Check sheet for the modelled part. Datum: model origin and axes. Units: mm. A direction names the side the tool comes from. Coordinates: 2 decimals unless noted, no trailing zeros. Loops run counter-clockwise (first coordinate to the right, second up) from the corner with the lowest first, then second, coordinate; pieces in that order, holes last. Notation, with made-up numbers: M -22,38.25 L 20,38.25 A31 cw 20,76.25 Z; hole C 15.5,-36 d10. An arc over 180 degrees is marked long. Answer in a Markdown table with one row per item. Add a question column.
```python
from build123d import *

# Parameters (mm, degrees)
SKETCH3_W            = 55.1053
SKETCH3_H            = 45.5803
BOSS_EXTRUDE2_DEPTH  = 44.45
SKETCH11_W           = 51.1175
SKETCH11_H           = 41.5925
SKETCH11_W_2         = 47.9425
SKETCH11_H_2         = 38.4175
BOSS_EXTRUDE3_DEPTH  = 3.175
SKETCH13_W           = 44.7675
SKETCH13_H           = 35.2425
CUT_EXTRUDE3_DEPTH   = 73.294764944
CUT_EXTRUDE4_DEPTH   = 5.1689
SKETCH19_W           = 1.5875
SKETCH19_H           = 45.5803
BOSS_EXTRUDE4_DEPTH  = 44.45
SKETCH21_W           = 1.905
SKETCH21_H           = 35.2425
CUT_EXTRUDE5_DEPTH   = 39.37
FILLET1_R            = 406.4
FILLET2_R            = 406.4
SKETCH22_R           = 1.524
CUT_EXTRUDE7_DEPTH   = 3.175
BOSS_EXTRUDE5_DEPTH  = 38.1
SKETCH39_R           = 1.296908885
SKETCH39_R_2         = 1.27
CUT_EXTRUDE14_DEPTH  = 25.4
BOSS_EXTRUDE22_DEPTH = 8.89
CUT_EXTRUDE15_DEPTH  = 88.778493945
SKETCH48_W           = 18.8595
SKETCH48_H           = 29.21
BOSS_EXTRUDE23_DEPTH = 1.5875
SKETCH52_R           = 1.27
CUT_EXTRUDE16_DEPTH  = 25.4


with BuildPart() as part:
    # Sketch3 → Boss-Extrude2 (new body)
    with BuildSketch(Plane(origin=(0, 0, 0), x_dir=(1, 0, 0), z_dir=(0, 1, 0))):
        with Locations((6.69887245, -22.79015)):
            Rectangle(SKETCH3_W, SKETCH3_H)
    extrude(amount=BOSS_EXTRUDE2_DEPTH)

    # Sketch11 → Boss-Extrude3 (add)
    with BuildSketch(Plane(origin=(0, 44.45, 0), x_dir=(1, 0, 0), z_dir=(0, 1, 0))):
        with Locations((6.69887245, -22.79015)):
            Rectangle(SKETCH11_W, SKETCH11_H)
        with Locations((6.69887245, -22.79015)):
            Rectangle(SKETCH11_W_2, SKETCH11_H_2, mode=Mode.SUBTRACT)
    extrude(amount=BOSS_EXTRUDE3_DEPTH)

    # Sketch13 → Cut-Extrude3 (cut, through all)
    with BuildSketch(Plane(origin=(0, 44.45, 0), x_dir=(1, 0, 0), z_dir=(0, 1, 0))):
        with Locations((6.69887245, -22.79015)):
            Rectangle(SKETCH13_W, SKETCH13_H)
    extrude(amount=-CUT_EXTRUDE3_DEPTH, mode=Mode.SUBTRACT)

    # Sketch14 → Cut-Extrude4 (cut)
    with BuildSketch(Plane.XY.offset(45.5803)):
        with BuildLine():
            Line((-2.82612755, 6.35), (-2.82612755, 0))
            Line((-2.82612755, 0), (3.52387245, 0))
            Line((3.52387245, 0), (3.52387245, 6.35))
            ThreePointArc((3.52387245, 6.35), (0.34887245, 9.525), (-2.82612755, 6.35))
        make_face()
        with BuildLine():
            Line((9.87387245, 6.35), (9.87387245, 0))
            Line((9.87387245, 0), (16.22387245, 0))
            Line((16.22387245, 0), (16.22387245, 6.35))
            ThreePointArc((16.22387245, 6.35), (13.04887245, 9.525), (9.87387245, 6.35))
        make_face()
        with BuildLine():
            Line((26.465313364, 0), (30.581222486, 0))
            Line((30.581222486, 0), (30.581222486, 6.35))
            ThreePointArc((30.581222486, 6.35), (28.523267925, 8.407954561), (26.465313364, 6.35))
            Line((26.465313364, 6.35), (26.465313364, 0))
        make_face()
    extrude(amount=-CUT_EXTRUDE4_DEPTH, mode=Mode.SUBTRACT)

    # Sketch19 → Boss-Extrude4 (add)
    with BuildSketch(Plane.XZ):
        with Locations((-21.64752755, 22.79015)):
            Rectangle(SKETCH19_W, SKETCH19_H)
        with Locations((35.04527245, 22.79015)):
            Rectangle(SKETCH19_W, SKETCH19_H)
    extrude(amount=-BOSS_EXTRUDE4_DEPTH)

    # Sketch21 → Cut-Extrude5 (cut)
    with BuildSketch(Plane(origin=(0, 0, 0), x_dir=(-1, 0, 0), z_dir=(0, -1, 0))):
        with Locations((16.63737755, -22.79015)):
            Rectangle(SKETCH21_W, SKETCH21_H)
        with Locations((-30.03512245, -22.79015)):
            Rectangle(SKETCH21_W, SKETCH21_H)
    extrude(amount=-CUT_EXTRUDE5_DEPTH, mode=Mode.SUBTRACT)

    # Fillet1
    # the kernel refuses this fillet: 406.4 mm, written as the material it adds along each edge
    with BuildSketch(Plane(origin=(-17.58987755, 39.37, 40.4114), x_dir=(0, -1, 0), z_dir=(0, 0, -1))) as fillet1_piece_1:
        with BuildLine():
            CenterArc((39.303371039, -406.4), FILLET1_R, 90, 5.549809332)
            Line((0, -1.905), (0, 0))
            Line((0, 0), (39.303371039, 0))
        make_face()
    extrude(amount=35.2425)

    # Fillet2
    # the kernel refuses this fillet: 406.4 mm, written as the material it adds along each edge
    with BuildSketch(Plane(origin=(30.98762245, 39.37, -93.089527597), x_dir=(-1, 0, 0), z_dir=(0, 0, 1))) as fillet2_piece_1_section:
        with BuildLine():
            CenterArc((406.4, 39.303371039), FILLET2_R, 180, 5.549809332)
            Line((0, 39.303371039), (0, 0))
            Line((0, 0), (1.905, 0))
        make_face()
    fillet2_piece_1 = extrude(amount=231.759355193, mode=Mode.PRIVATE)
    fillet2_piece_1 = split(fillet2_piece_1, bisect_by=Plane(origin=(30.98762245, 39.37, 45.5803), z_dir=(0, 0, -1)), keep=Keep.TOP, mode=Mode.PRIVATE)
    fillet2_piece_1 = split(fillet2_piece_1, bisect_by=Plane(origin=(30.98762245, 39.37, 0), z_dir=(0, 0, 1)), keep=Keep.TOP, mode=Mode.PRIVATE)
    add(fillet2_piece_1)

    # Sketch22 → Cut-Extrude7 (cut)
    with BuildSketch(Plane.XZ):
        with Locations(Location((-19.64727755, 42.7863, 0), (0, 0, 270))):
            Circle(SKETCH22_R)
        with Locations(Location((33.04502245, 42.7863, 0), (0, 0, 270))):
            Circle(SKETCH22_R)
        with Locations(Location((-19.64727755, 2.794, 0), (0, 0, 270))):
            Circle(SKETCH22_R)
        with Locations(Location((33.04502245, 2.794, 0), (0, 0, 270))):
            Circle(SKETCH22_R)
    extrude(amount=-CUT_EXTRUDE7_DEPTH, mode=Mode.SUBTRACT)

    # Sketch23 → Boss-Extrude5 (add)
    with BuildSketch(Plane.XZ):
        with BuildLine():
            Line((22.13572245, 62.8523), (22.13572245, 64.4398))
            Line((22.13572245, 64.4398), (21.379894456, 64.4398))
            Line((21.379894456, 64.4398), (-12.40827755, 64.4398))
            add(Edge.make_bspline(
                [(-12.40827755, 64.4398), (-22.44127755, 64.4398), (-22.44127755, 45.5803)],
                knots=[0, 0, 0, 1.570796327, 1.570796327, 1.570796327], degree=2, weights=[1, 0.707106781, 1]))
            Line((-22.44127755, 45.5803), (-11.13827755, 45.5803))
            Line((-11.13827755, 45.5803), (-11.13827755, 58.170091836))
            Line((-11.13827755, 58.170091836), (-11.13827755, 62.8523))
            Line((-11.13827755, 62.8523), (22.13572245, 62.8523))
        make_face()
    extrude(amount=-BOSS_EXTRUDE5_DEPTH)

    # Sketch39 → Cut-Extrude14 (cut)
    with BuildSketch(Plane.XY.offset(64.4398)):
        with Locations((5.46697245, 34.925)):
            Circle(SKETCH39_R)
        with Locations((-10.02702755, 34.925)):
            Circle(SKETCH39_R_2)
        with Locations((20.96097245, 34.925)):
            Circle(SKETCH39_R_2)
    extrude(amount=-CUT_EXTRUDE14_DEPTH, mode=Mode.SUBTRACT)

    # Sketch43 → Boss-Extrude22 (add)
    with BuildSketch(Plane.XZ):
        with BuildLine():
            Line((30.58122245, 45.5803), (35.83902245, 45.5803))
            add(Edge.make_bspline(
                [(35.83902245, 45.5803), (35.83902245, 63.254133988), (24.53602245, 64.4398)],
                knots=[4.71238898, 4.71238898, 4.71238898, 6.216048931, 6.216048931, 6.216048931], degree=2, weights=[1, 0.730440262, 1]))
            Line((24.53602245, 64.4398), (22.13572245, 64.4398))
            Line((22.13572245, 64.4398), (22.13572245, 45.5803))
            Line((22.13572245, 45.5803), (23.72322245, 45.5803))
            Line((23.72322245, 45.5803), (23.72322245, 58.7883))
            Line((23.72322245, 58.7883), (30.58122245, 58.7883))
            Line((30.58122245, 58.7883), (30.58122245, 45.5803))
        make_face()
    extrude(amount=-BOSS_EXTRUDE22_DEPTH)

    # Sketch51 → Cut-Extrude15 (cut, through all)
    with BuildSketch(Plane.XY.offset(64.4398)):
        with BuildLine():
            add(Edge.make_bspline(
                [(-20.85377755, 44.45), (-22.44127755, 44.45), (-22.44127755, 8.89)],
                knots=[3.141592654, 3.141592654, 3.141592654, 4.71238898, 4.71238898, 4.71238898], degree=2, weights=[1, 0.707106781, 1]))
            Line((-22.44127755, 8.89), (-23.728758276, 8.89))
            Line((-23.728758276, 8.89), (-23.728758276, 45.620970636))
            Line((-23.728758276, 45.620970636), (-20.85377755, 45.620970636))
            Line((-20.85377755, 45.620970636), (-20.85377755, 44.45))
        make_face()
        with BuildLine():
            add(Edge.make_bspline(
                [(35.83902245, 8.89), (35.83902245, 34.352534387), (34.251533964, 44.439253731)],
                knots=[4.71238898, 4.71238898, 4.71238898, 5.875876601, 5.875876601, 5.875876601], degree=2, weights=[1, 0.835505729, 1]))
            Line((34.251533964, 44.439253731), (34.25152245, 44.45))
            Line((34.25152245, 44.45), (34.25152245, 45.620970636))
            Line((34.25152245, 45.620970636), (37.555875031, 45.620970636))
            Line((37.555875031, 45.620970636), (37.555875031, 8.89))
            Line((37.555875031, 8.89), (35.83902245, 8.89))
        make_face()
    extrude(amount=-CUT_EXTRUDE15_DEPTH, mode=Mode.SUBTRACT)

    # Sketch48 → Boss-Extrude23 (add)
    with BuildSketch(Plane(origin=(22.13572245, 0, 0), x_dir=(0, 0, -1), z_dir=(1, 0, 0))):
        with Locations((-55.01005, 23.495)):
            Rectangle(SKETCH48_W, SKETCH48_H)
    extrude(amount=BOSS_EXTRUDE23_DEPTH)

    # Sketch52 → Cut-Extrude16 (cut)
    with BuildSketch(Plane.XY.offset(64.4398)):
        with Locations((20.96097245, 34.925)):
            Circle(SKETCH52_R)
    extrude(amount=-CUT_EXTRUDE16_DEPTH, mode=Mode.SUBTRACT)


solid = part.part
```
Q1. Thickness scan on L1, parallel to Z at x = 8.5, y = 5; L2, parallel to Z at x = -12, y = 38; L3, parallel to Z at x = 9.5, y = 41. Record the ranges inside material, lowest first.
Q2. Cross-section at B-B (x = 5). Record the cut outline in (y, z) (3 decimals), plus the area to 3 significant figures.
Q3. Go/stop test with flat-tipped pins: pin 1 (0.9 mm diameter, centred on x = 32.5, z = 43.5, fed in from -Y) (3 decimals); pin 2 (20.5 mm diameter, centred on y = 13.5, z = 58, fed in from +X); pin 3 (3 mm diameter, centred on y = 20.5, z = 49, fed in from +X). Record where each tip stops, or that it passes through.
Q4. Mould release check, pull along Z, two halves, no side actions. Record for faces 1 (the face through (-19.19, 1.565, 41.333)), 2 (the face through (5, 47.625, 43)), 3 (the face through (22.136, 37, 54)): released by +Z, released by -Z, zero draft, split by the parting line, or undercut.
Q5. Cross-section at C-C (z = 57). Count the separate pieces of the cut face and the enclosed holes in it, plus the area to 3 significant figures.
Q6. Cross-section at A-A (x = 11.5). Record the cut outline in (y, z) (3 decimals), plus the area to 3 significant figures.
Q7. Access from +Z, -Z, +X, -X, +Y, -Y to the whole of each face (thin tool, end or side, straight path). Record for faces 4 (the face through (-13, 38.1, 56)), 5 (the face through (7, 0, 43)), 6 (the face through (13.119, 9.524, 43.032)), 7 (the face through (6, 46, 3.581)), 8 (the face through (-11.138, 37, 54)).
Answer key:
| question | item | result |
|---|---|---|
| 1 | L1 | 0 to 5.17, 40.41 to 45.58, 62.85 to 64.44 |
| 1 | L2 | 0 to 5.17, 40.41 to 64.44 |
| 1 | L3 | 0 to 5.17, 40.41 to 45.58 |
| 2 | outline | M 0,0 L 44.45,0 L 44.45,1.994 L 47.625,1.994 L 47.625,3.581 L 44.45,3.581 L 44.45,5.169 L 0,5.169 Z; M 0,40.411 L 33.715,40.411 L 33.715,45.58 L 0,45.58 Z; M 0,62.852 L 33.715,62.852 L 33.715,64.44 L 0,64.44 Z; M 36.135,40.411 L 44.45,40.411 L 44.45,41.999 L 47.625,41.999 L 47.625,43.586 L 44.45,43.586 L 44.45,45.58 L 36.135,45.58 Z; M 36.135,62.852 L 38.1,62.852 L 38.1,64.44 L 36.135,64.44 Z |
| 2 | area | 514 mm^2 |
| 3 | pin 1 | y = 3.175 |
| 3 | pin 2 | x = 35.66 |
| 3 | pin 3 | x = 23.72 |
| 4 | face 1 | undercut |
| 4 | face 2 | zero draft |
| 4 | face 3 | undercut |
| 5 | separate pieces | 3 |
| 5 | enclosed holes | 0 |
| 5 | area | 438 mm^2 |
| 6 | outline | M 0,0 L 44.45,0 L 44.45,1.994 L 47.625,1.994 L 47.625,3.581 L 44.45,3.581 L 44.45,5.169 L 0,5.169 Z; M 0,62.852 L 38.1,62.852 L 38.1,64.44 L 0,64.44 Z; M 9.122,40.411 L 44.45,40.411 L 44.45,41.999 L 47.625,41.999 L 47.625,43.586 L 44.45,43.586 L 44.45,45.58 L 9.122,45.58 Z |
| 6 | area | 483 mm^2 |
| 7 | face 4 | +Z, +X, -X, +Y |
| 7 | face 5 | +Z, -Z, +X, -X, -Y |
| 7 | face 6 | -Y |
| 7 | face 7 | +Y |
| 7 | face 8 | +Y, -Y |
